```python
from build123d import *

# Parameters (mm, degrees)
SKETCH1_W           = 44
SKETCH1_H           = 44
BOSS_EXTRUDE1_DEPTH = 10
BOSS_EXTRUDE2_DEPTH = 12.7
SKETCH3_R           = 2.6
CUT_EXTRUDE1_DEPTH  = 63.929245983
SKETCH4_R           = 4.275
CUT_EXTRUDE2_DEPTH  = 66.177373375
FILLET1_R           = 3
FILLET2_R           = 5
FILLET3_R           = 0.5


with BuildPart() as part:
    # Sketch1 → Boss-Extrude1 (new body)
    with BuildSketch(Plane.XY):
        Rectangle(SKETCH1_W, SKETCH1_H)
        with BuildLine():
            Line((7, 12), (-7, 12))
            ThreePointArc((-7, 12), (-10.535533906, 10.535533906), (-12, 7))
            Line((-12, 7), (-12, -7))
            ThreePointArc((-12, -7), (-10.535533906, -10.535533906), (-7, -12))
            Line((-7, -12), (7, -12))
            ThreePointArc((7, -12), (10.535533906, -10.535533906), (12, -7))
            Line((12, -7), (12, 7))
            ThreePointArc((12, 7), (10.535533906, 10.535533906), (7, 12))
        make_face(mode=Mode.SUBTRACT)
        with BuildLine():
            Line((-19, 17.2), (-12, 17.2))
            ThreePointArc((-12, 17.2), (-10.25, 15.45), (-12, 13.7))
            Line((-12, 13.7), (-19, 13.7))
            ThreePointArc((-19, 13.7), (-20.75, 15.45), (-19, 17.2))
        make_face(mode=Mode.SUBTRACT)
        with BuildLine():
            Line((-19, -17.2), (-12, -17.2))
            ThreePointArc((-12, -17.2), (-10.25, -15.45), (-12, -13.7))
            Line((-12, -13.7), (-19, -13.7))
            ThreePointArc((-19, -13.7), (-20.75, -15.45), (-19, -17.2))
        make_face(mode=Mode.SUBTRACT)
        with BuildLine():
            Line((12, 17.2), (19, 17.2))
            ThreePointArc((19, 17.2), (20.75, 15.45), (19, 13.7))
            Line((19, 13.7), (12, 13.7))
            ThreePointArc((12, 13.7), (10.25, 15.45), (12, 17.2))
        make_face(mode=Mode.SUBTRACT)
        with BuildLine():
            Line((12, -13.7), (19, -13.7))
            ThreePointArc((19, -13.7), (20.75, -15.45), (19, -17.2))
            Line((19, -17.2), (12, -17.2))
            ThreePointArc((12, -17.2), (10.25, -15.45), (12, -13.7))
        make_face(mode=Mode.SUBTRACT)
    extrude(amount=BOSS_EXTRUDE1_DEPTH)

    # Sketch2 → Boss-Extrude2 (add)
    with BuildSketch(Plane(origin=(22, 0, 0), x_dir=(0, 0, -1), z_dir=(1, 0, 0))):
        Polygon((0, 12), (-40, 12), (-40, 16), (-40, 22), (-10, 22), (0, 22), align=None)
    boss_extrude2 = extrude(amount=BOSS_EXTRUDE2_DEPTH)

    # Sketch3 → Cut-Extrude1 (cut, through all)
    with BuildSketch(Plane.XZ.offset(-12)):
        with Locations((28.6, 35)):
            Circle(SKETCH3_R)
        with Locations((28.6, 9)):
            Circle(SKETCH3_R)
    cut_extrude1 = extrude(amount=-CUT_EXTRUDE1_DEPTH, mode=Mode.SUBTRACT)

    # Sketch4 → Cut-Extrude2 (cut, through all)
    with BuildSketch(Plane(origin=(0, 16, 0), x_dir=(-1, 0, 0), z_dir=(0, -1, 0))):
        with Locations(Location((-28.6, -9, 0), (0, 0, 180))):
            Circle(SKETCH4_R)
        with Locations(Location((-28.6, -35, 0), (0, 0, 180))):
            Circle(SKETCH4_R)
    cut_extrude2 = extrude(amount=-CUT_EXTRUDE2_DEPTH, mode=Mode.SUBTRACT)

    # Mirror1: Boss-Extrude2, Cut-Extrude1, Cut-Extrude2 across plane
    add(boss_extrude2.mirror(Plane(origin=(0, 0, 0), x_dir=(0, 0, 1), z_dir=(1, 0, 0))))
    add(cut_extrude1.mirror(Plane(origin=(0, 0, 0), x_dir=(0, 0, 1), z_dir=(1, 0, 0))), mode=Mode.SUBTRACT)
    add(cut_extrude2.mirror(Plane(origin=(0, 0, 0), x_dir=(0, 0, 1), z_dir=(1, 0, 0))), mode=Mode.SUBTRACT)

    # Fillet1
    fillet1_edges = [part.edges().sort_by_distance(p)[0] for p in [
        (34.7, 17, 0),
        (34.7, 17, 40),
        (-34.7, 17, 0),
        (-34.7, 17, 40),
        (-22, 17, 40),
        (22, 17, 40),
    ]]
    fillet(fillet1_edges, radius=FILLET1_R)

    # Fillet2
    fillet2_edges = [part.edges().sort_by_distance(p)[0] for p in [
        (22, -22, 5),
        (-22, -22, 5),
    ]]
    fillet(fillet2_edges, radius=FILLET2_R)

    # Fillet3
    fillet3_edges = [part.edges().sort_by_distance(p)[0] for p in [
        (-22, 17, 10),
        (22, 17, 10),
    ]]
    fillet(fillet3_edges, radius=FILLET3_R)


solid = part.part
```
Could you check a few things on this model? Use its own coordinates, in mm. A direction names the side the tool comes from. Give positions to 0.01 mm unless a question says otherwise; leave off trailing zeros. Order: outer loops, then holes, each group sorted by start corner. A loop starts at its lowest first (then second) coordinate and runs counter-clockwise, first axis right, second up.
Q1. Suppose I cut it at C-C, the plane y = -6. Write out the boundary of the cut face in (x, z).
Q2. For faces 4 (the flat face through (-22, -3, 5)), 5 (the cylindrical face through (-10.25, 15.49, 4.93)), 6 (the flat face through (22, -3, 5)), 7 (the cylindrical face through (-32.68, 18.96, 10.28)), which set-ups out of +Z, -Z, +X, -X, +Y, -Y let a thin tool reach every point of the face, with its end or its side?
Q3. Suppose I cut it at A-A, the plane y = -15.45. Write out the boundary of the cut face in (x, z).
Q4. If I drill on line 1 along Z through (x, y) = (-28.6, 14.5); line 2 along Z through (x, y) = (-28.6, 17.8) (3 decimals); line 3 along Y through (x, z) = (-13.5, 6), over which ranges is the centre line in solid material (lowest first)?
Q5. I'm going to push flat-ended pins straight in: P1, Ø7, axis at x = -29, z = 9, coming from the +Y side; P2, Ø10.5, axis at x = 27, z = 29.5, coming from the -Y side; P3, Ø3, axis at y = 2.5, z = 6.5, coming from the -X side; P4, Ø7, axis at x = -27, z = 33.5, coming from the +Y side. Where does each tip first touch, or does it pass through?
Q6. We'd pull the mould along Z, two halves only. Please class faces 1 (the flat face through (-15, -13.7, 5)), 2 (the flat face through (0, 15, 0)), 3 (the cylindrical face through (31, 14, 8)): +Z half, -Z half, draft (parallel to the pull), parting line (faces both ways), or undercut.
Q7. Suppose I cut it at B-B, the plane z = 26. Write out the boundary of the cut face in (x, y), and give its area (3 significant figures).
Q8. Suppose I cut it at D-D, the plane z = 7.5. Count the separate pieces of the cut face and the enclosed holes in it, and give its area (3 significant figures).
Solution:
1. outline: (-22, 0) - (-12, 0) - (-12, 10) - (-22, 10) - close; (12, 0) - (22, 0) - (22, 10) - (12, 10) - close
2. face 4: +Z, -Z, -X, -Y
2. face 5: +Z, -Z
2. face 6: +Z, -Z, +X, -Y
2. face 7: +Y
3. outline: (-22, 0) - (-20.75, 0) - (-20.75, 10) - (-22, 10) - close; (-10.25, 0) - (10.25, 0) - (10.25, 10) - (-10.25, 10) - close; (20.75, 0) - (22, 0) - (22, 10) - (20.75, 10) - close
4. line 1: z = 0 to 6.4, 11.6 to 32.4, 37.6 to 40
4. line 2: z = 0 to 4.725, 13.275 to 30.725, 39.275 to 40
4. line 3: y = -22 to -17.2, -13.7 to 13.7, 17.2 to 22
5. P1: stops at y = 16
5. P2: stops at y = 12
5. P3: stops at x = -22
5. P4: stops at y = 22
6. face 1: draft
6. face 2: -Z half
6. face 3: undercut
7. outline: (-34.7, 12) - (-22, 12) - (-22, 22) - (-34.7, 22) - close; (22, 12) - (34.7, 12) - (34.7, 22) - (22, 22) - close
7. area: 254 mm2
8. separate pieces: 3
8. enclosed holes: 5
8. area: 1,360 mm2
